```python
from build123d import *

# Parameters (mm, degrees)
F1_DEPTH = 25.4
F3_D     = 4.2


with BuildPart() as f1:
    # F0 (on Top) → F1 (new body)
    with BuildSketch(Plane.XY):
        Polygon((75.6428092718, -74.5307654142), (75.6428092718, 0), (75.6428092718, 76.6944885254), (-76.9004449248, 76.6944885254), (-76.9004449248, -74.5307654142), align=None)
    extrude(amount=-F1_DEPTH)

    # F3 (through all)
    with Locations(Plane.XY):
        with Locations((0, 0)):
            Hole(F3_D / 2)


solid = f1.part
```
Can you work these out from the model? Positions are in its coordinate system, mm. Coordinates: 2 decimals unless noted, no trailing zeros. Write each loop counter-clockwise with the first axis right and the second up, starting at its lowest first coordinate (ties: lowest second). Pieces come first, ordered by that corner, then holes. Notation, with made-up numbers: (56.25, -14) - (74.25, -14) arc R20 cw to (74.25, 13) - close; hole circle Ø7 at (22.5, 23.25). An arc over 180 degrees is marked (long way). Return JSON: item names as keys, results as strings.
Q1. Please list where these lines run through material, in increasing order: L1, parallel to Y at x = 0, z = -8.75; L2, parallel to X at y = -0.5, z = -6.25; L3, parallel to Y at x = 0.5, z = -11.5. Write a range as from..to.
Computed values:
{"L1": "y = -74.53..-2.1, 2.1..76.69", "L2": "x = -76.9..-2.04, 2.04..75.64", "L3": "y = -74.53..-2.04, 2.04..76.69"}
Q2. Thinking about a two-plate mould opening in Y: for faces 1 (the flat face through (-76.9, 2, -13)), 2 (the flat face through (0, 76.694, -13)), 3 (the cylindrical face through (-2.003, 0.631, -12.878)), which applies, +Y half, -Y half, draft (parallel to the pull), parting line (faces both ways), or undercut?
Computed values:
{"face 1": "draft", "face 2": "+Y half", "face 3": "undercut"}
Q3. If we section it at B-B (y = 0): Please give me the cut outline in (x, z).
Computed values:
{"outline": "(-76.9, -25.4) - (-2.1, -25.4) - (-2.1, 0) - (-76.9, 0) - close; (2.1, -25.4) - (75.64, -25.4) - (75.64, 0) - (2.1, 0) - close"}
Q4. If we section it at A-A (x = 0): Please give me the cut outline in (y, z), then the cut area to 3 significant figures.
Computed values:
{"outline": "(-74.53, -25.4) - (-2.1, -25.4) - (-2.1, 0) - (-74.53, 0) - close; (2.1, -25.4) - (76.69, -25.4) - (76.69, 0) - (2.1, 0) - close", "area": "3,730 mm2"}
Q5. I'm going to push a flat-ended pin straight in: pin 1 Ø3.5 at (x, y) = (0, 0) entering from +Z. Where does the tip first touch, or does it pass through?
Computed values:
{"pin 1": "passes through"}
